Can you work these out from the drawing? Everything is in mm from the part's minimum corner. Round coordinates to 2 decimals unless told otherwise and drop trailing zeros. Order: outer loops, then holes, each group sorted by start corner. A loop starts at its lowest first (then second) coordinate and runs counter-clockwise, first axis right, second up. Notation, with made-up numbers: (14, 26.25) - (52, 26.25) arc R16 ccw to (52, 38.25) - close; hole circle Ø1 at (-7, 86.5). An arc over 180 degrees is marked (long way). Answer as a JSON object with one key per item and string values.
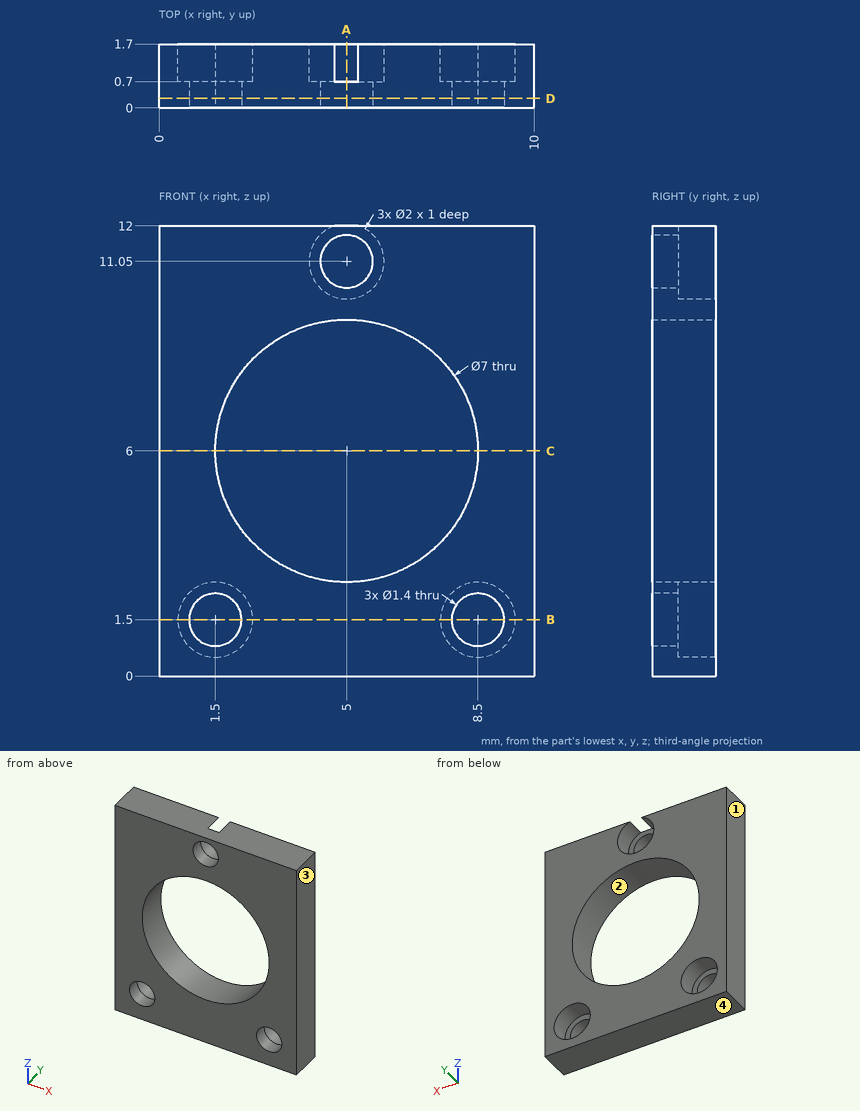
1. Imagine slicing it at D-D (y = 0.25). List the corners of the cut face in (x, z) for me.
Responses:
{"outline": "(0, 0) - (10, 0) - (10, 12) - (0, 12) - close; hole circle Ø1.4 at (1.5, 1.5); hole circle Ø7 at (5, 6); hole circle Ø1.4 at (5, 11.05); hole circle Ø1.4 at (8.5, 1.5)"}
2. Thinking about a two-plate mould opening in X: for the marked faces 1, 2, 3 and 4, which applies, pulls with the +X half, pulls with the -X half, needs draft (parallel to the pull), parting line crosses it, or undercut?
Responses:
{"face 1": "pulls with the -X half", "face 2": "undercut", "face 3": "pulls with the +X half", "face 4": "needs draft"}
3. Imagine slicing it at A-A (x = 5). List the corners of the cut face in (y, z) for me.
Responses:
{"outline": "(0, 0) - (1.7, 0) - (1.7, 2.5) - (0, 2.5) - close; (0, 9.5) - (1.7, 9.5) - (1.7, 10.05) - (0.7, 10.05) - (0.7, 10.35) - (0, 10.35) - close; (0, 11.75) - (0.7, 11.75) - (0.7, 12) - (0, 12) - close"}
4. If I drill on L1, parallel to X at y = 1.3, z = 1.5; L2, parallel to Z at x = 8, y = 1.55; L3, parallel to X at y = 1.55, z = 6.5, over which ranges is the centre line in solid material (lowest first)? Write a range as [from, to].
Responses:
{"L1": "[0, 0.5], [2.5, 7.5], [9.5, 10]", "L2": "[0, 0.63], [2.37, 4.2], [7.8, 12]", "L3": "[0, 1.54], [8.46, 10]"}
5. Imagine slicing it at B-B (z = 1.5). List the corners of the cut face in (x, y) for me.
Responses:
{"outline": "(0, 0) - (0.8, 0) - (0.8, 0.7) - (0.5, 0.7) - (0.5, 1.7) - (0, 1.7) - close; (2.2, 0) - (7.8, 0) - (7.8, 0.7) - (7.5, 0.7) - (7.5, 1.7) - (2.5, 1.7) - (2.5, 0.7) - (2.2, 0.7) - close; (9.2, 0) - (10, 0) - (10, 1.7) - (9.5, 1.7) - (9.5, 0.7) - (9.2, 0.7) - close"}
6. For P1, Ø1.8, axis at x = 1.5, z = 1.5, coming from the +Y side; P2, Ø1.2, axis at x = 8.5, z = 1.5, coming from the -Y side, each with a flat end and sliding along its axis, tell me the tip position at first contact or that it passes through.
Responses:
{"P1": "y = 0.7", "P2": "through"}
7. Imagine slicing it at C-C (z = 6). List the corners of the cut face in (x, y) for me, plus the area to 3 significant figures.
Responses:
{"outline": "(0, 0) - (1.5, 0) - (1.5, 1.7) - (0, 1.7) - close; (8.5, 0) - (10, 0) - (10, 1.7) - (8.5, 1.7) - close", "area": "5.10 mm2"}
